Input: dimensioned drawing with shaded views. Units: mm. Origin: part minimum x, y, z. A direction names the side the tool comes from. Give positions to 0.01 mm unless a question says otherwise; leave off trailing zeros. Loops run counter-clockwise (first coordinate to the right, second up) from the corner with the lowest first, then second, coordinate; pieces in that order, holes last. Notation, with made-up numbers: (82, 70) -> (86, 70) arc R18 cw to (86, 101) -> close; hole circle Ø11 at (0, 83). An arc over 180 degrees is marked (long way). One line per question, with ' | ' between items. Start each with the question number.
Item 1: Section B-B on x = 12. Return loops of the section in (y, z), then the cut area to 3 significant figures.
Item 2: Section A-A on z = 39. Return loops of the section in (x, y), then the cut area to 3 significant figures.
Item 3: Material intervals for line 1 along Z through (x, y) = (10.25, 5.5); line 2 along Y through (x, z) = (19.5, 14); line 3 along Z through (x, y) = (20.5, 6.25), sorted ascending. Write a range as [from, to].
Item 4: Pin query (flat end, axial travel): P1, Ø12.5, axis at x = 17, z = 23.5, coming from the +Y side; P2, Ø2, axis at x = 20, y = 0.5, coming from the -Z side; P3, Ø0.6, axis at x = 2.5, y = 0.5, coming from the -Z side. Return the tip coordinate at first contact, or that it passes through.
Item 5: Section C-C on z = 25.5. Return loops of the section in (x, y).
Item 6: Section D-D on x = 5.5. Return loops of the section in (y, z).
Item 7: Set-up query: the marked faces 1 and 2. Return all of +Z, -Z, +X, -X, +Y, -Y with unobstructed straight access to the full face (end or side cutting, diameter ignored); none if empty.
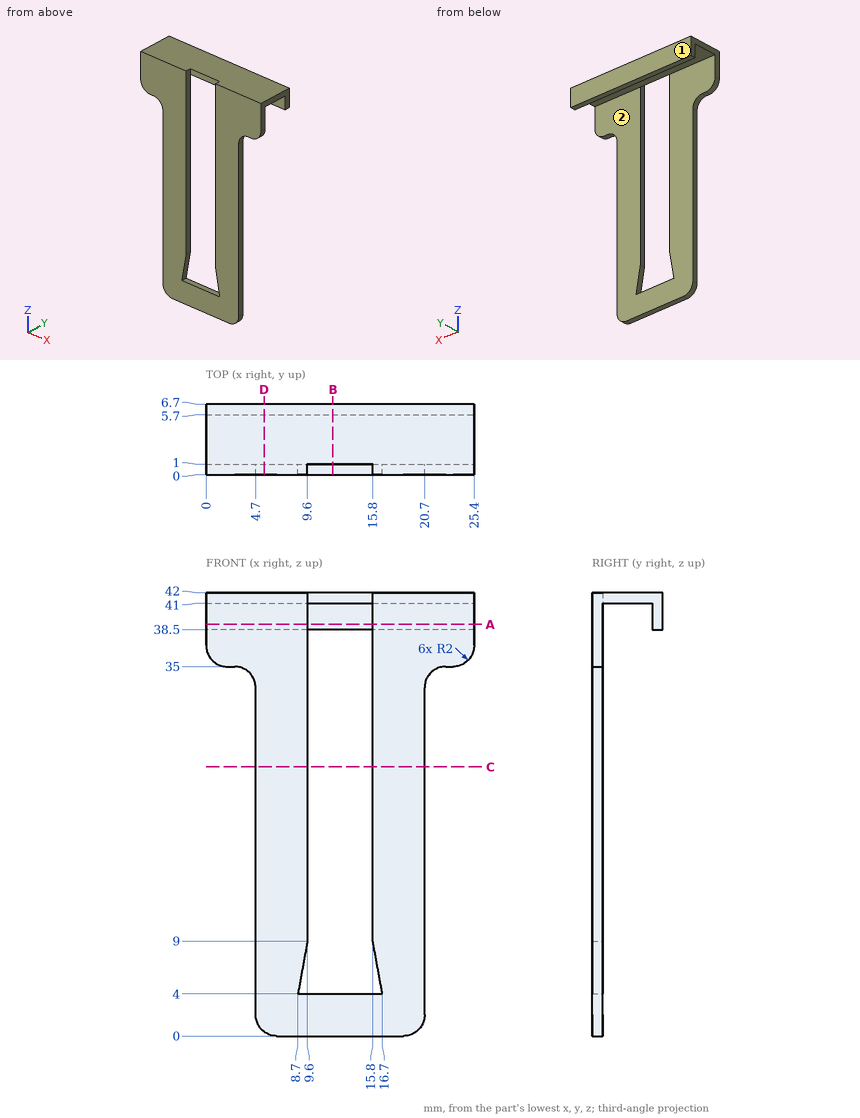
Result sheet:
1) outline: (0, 0) -> (1, 0) -> (1, 4) -> (0, 4) -> close; (1, 41) -> (5.7, 41) -> (5.7, 38.5) -> (6.7, 38.5) -> (6.7, 42) -> (1, 42) -> close | area: 12.2 mm²
2) outline: (0, 0) -> (9.6, 0) -> (9.6, 1) -> (0, 1) -> close; (0, 5.7) -> (25.4, 5.7) -> (25.4, 6.7) -> (0, 6.7) -> close; (15.8, 0) -> (25.4, 0) -> (25.4, 1) -> (15.8, 1) -> close | area: 44.6 mm²
3) line 1: z = [41, 42] | line 2: y = [0, 1] | line 3: z = [38.5, 42]
4) P1: stops at y = 1 | P2: stops at z = 0.02 | P3: stops at z = 35
5) outline: (4.7, 0) -> (9.6, 0) -> (9.6, 1) -> (4.7, 1) -> close; (15.8, 0) -> (20.7, 0) -> (20.7, 1) -> (15.8, 1) -> close
6) outline: (0, 0.4) -> (1, 0.4) -> (1, 41) -> (5.7, 41) -> (5.7, 38.5) -> (6.7, 38.5) -> (6.7, 42) -> (0, 42) -> close
7) face 1: +Z, -Z, +X, -X, +Y | face 2: -Z, +X, -X
